```python
from build123d import *

# Parameters (mm, degrees)
SKETCH1_W           = 50.8
SKETCH1_H           = 304.8
BOSS_EXTRUDE1_DEPTH = 6.35
SKETCH2_R           = 3.429
CUT_EXTRUDE1_DEPTH  = 310.0695755


with BuildPart() as part:
    # Sketch1 → Boss-Extrude1 (new body)
    with BuildSketch(Plane.XY):
        with Locations((25.4, -152.4)):
            Rectangle(SKETCH1_W, SKETCH1_H)
    extrude(amount=BOSS_EXTRUDE1_DEPTH)

    # Sketch2 → Cut-Extrude1 (cut, through all)
    with BuildSketch(Plane.XY):
        with Locations((6.35, -6.35)):
            Circle(SKETCH2_R)
        with Locations((19.05, -6.35)):
            Circle(SKETCH2_R)
        with Locations((31.75, -6.35)):
            Circle(SKETCH2_R)
        with Locations((44.45, -6.35)):
            Circle(SKETCH2_R)
        with Locations((19.05, -19.05)):
            Circle(SKETCH2_R)
        with Locations((31.75, -19.05)):
            Circle(SKETCH2_R)
        with Locations((44.45, -19.05)):
            Circle(SKETCH2_R)
        with Locations((19.05, -31.75)):
            Circle(SKETCH2_R)
        with Locations((31.75, -31.75)):
            Circle(SKETCH2_R)
        with Locations((44.45, -31.75)):
            Circle(SKETCH2_R)
        with Locations((19.05, -44.45)):
            Circle(SKETCH2_R)
        with Locations((31.75, -44.45)):
            Circle(SKETCH2_R)
        with Locations((44.45, -44.45)):
            Circle(SKETCH2_R)
        with Locations((19.05, -57.15)):
            Circle(SKETCH2_R)
        with Locations((31.75, -57.15)):
            Circle(SKETCH2_R)
        with Locations((44.45, -57.15)):
            Circle(SKETCH2_R)
        with Locations((19.05, -69.85)):
            Circle(SKETCH2_R)
        with Locations((31.75, -69.85)):
            Circle(SKETCH2_R)
        with Locations((44.45, -69.85)):
            Circle(SKETCH2_R)
        with Locations((19.05, -82.55)):
            Circle(SKETCH2_R)
        with Locations((31.75, -82.55)):
            Circle(SKETCH2_R)
        with Locations((44.45, -82.55)):
            Circle(SKETCH2_R)
        with Locations((19.05, -95.25)):
            Circle(SKETCH2_R)
        with Locations((31.75, -95.25)):
            Circle(SKETCH2_R)
        with Locations((44.45, -95.25)):
            Circle(SKETCH2_R)
        with Locations((19.05, -107.95)):
            Circle(SKETCH2_R)
        with Locations((31.75, -107.95)):
            Circle(SKETCH2_R)
        with Locations((44.45, -107.95)):
            Circle(SKETCH2_R)
        with Locations((19.05, -120.65)):
            Circle(SKETCH2_R)
        with Locations((31.75, -120.65)):
            Circle(SKETCH2_R)
        with Locations((44.45, -120.65)):
            Circle(SKETCH2_R)
        with Locations((19.05, -133.35)):
            Circle(SKETCH2_R)
        with Locations((31.75, -133.35)):
            Circle(SKETCH2_R)
        with Locations((44.45, -133.35)):
            Circle(SKETCH2_R)
        with Locations((19.05, -146.05)):
            Circle(SKETCH2_R)
        with Locations((31.75, -146.05)):
            Circle(SKETCH2_R)
        with Locations((44.45, -146.05)):
            Circle(SKETCH2_R)
        with Locations((19.05, -158.75)):
            Circle(SKETCH2_R)
        with Locations((31.75, -158.75)):
            Circle(SKETCH2_R)
        with Locations((44.45, -158.75)):
            Circle(SKETCH2_R)
        with Locations((19.05, -171.45)):
            Circle(SKETCH2_R)
        with Locations((31.75, -171.45)):
            Circle(SKETCH2_R)
        with Locations((44.45, -171.45)):
            Circle(SKETCH2_R)
        with Locations((19.05, -184.15)):
            Circle(SKETCH2_R)
        with Locations((31.75, -184.15)):
            Circle(SKETCH2_R)
        with Locations((44.45, -184.15)):
            Circle(SKETCH2_R)
        with Locations((19.05, -196.85)):
            Circle(SKETCH2_R)
        with Locations((31.75, -196.85)):
            Circle(SKETCH2_R)
        with Locations((44.45, -196.85)):
            Circle(SKETCH2_R)
        with Locations((19.05, -209.55)):
            Circle(SKETCH2_R)
        with Locations((31.75, -209.55)):
            Circle(SKETCH2_R)
        with Locations((44.45, -209.55)):
            Circle(SKETCH2_R)
        with Locations((19.05, -222.25)):
            Circle(SKETCH2_R)
        with Locations((31.75, -222.25)):
            Circle(SKETCH2_R)
        with Locations((44.45, -222.25)):
            Circle(SKETCH2_R)
        with Locations((19.05, -234.95)):
            Circle(SKETCH2_R)
        with Locations((31.75, -234.95)):
            Circle(SKETCH2_R)
        with Locations((44.45, -234.95)):
            Circle(SKETCH2_R)
        with Locations((19.05, -247.65)):
            Circle(SKETCH2_R)
        with Locations((31.75, -247.65)):
            Circle(SKETCH2_R)
        with Locations((44.45, -247.65)):
            Circle(SKETCH2_R)
        with Locations((19.05, -260.35)):
            Circle(SKETCH2_R)
        with Locations((31.75, -260.35)):
            Circle(SKETCH2_R)
        with Locations((44.45, -260.35)):
            Circle(SKETCH2_R)
        with Locations((19.05, -273.05)):
            Circle(SKETCH2_R)
        with Locations((31.75, -273.05)):
            Circle(SKETCH2_R)
        with Locations((44.45, -273.05)):
            Circle(SKETCH2_R)
        with Locations((19.05, -285.75)):
            Circle(SKETCH2_R)
        with Locations((31.75, -285.75)):
            Circle(SKETCH2_R)
        with Locations((44.45, -285.75)):
            Circle(SKETCH2_R)
        with Locations((19.05, -298.45)):
            Circle(SKETCH2_R)
        with Locations((31.75, -298.45)):
            Circle(SKETCH2_R)
        with Locations((44.45, -298.45)):
            Circle(SKETCH2_R)
        with Locations((19.05, -311.15)):
            Circle(SKETCH2_R)
        with Locations((31.75, -311.15)):
            Circle(SKETCH2_R)
        with Locations((44.45, -311.15)):
            Circle(SKETCH2_R)
        with Locations((19.05, -323.85)):
            Circle(SKETCH2_R)
        with Locations((31.75, -323.85)):
            Circle(SKETCH2_R)
        with Locations((44.45, -323.85)):
            Circle(SKETCH2_R)
        with Locations((19.05, -336.55)):
            Circle(SKETCH2_R)
        with Locations((31.75, -336.55)):
            Circle(SKETCH2_R)
        with Locations((44.45, -336.55)):
            Circle(SKETCH2_R)
        with Locations((19.05, -349.25)):
            Circle(SKETCH2_R)
        with Locations((31.75, -349.25)):
            Circle(SKETCH2_R)
        with Locations((44.45, -349.25)):
            Circle(SKETCH2_R)
        with Locations((19.05, -361.95)):
            Circle(SKETCH2_R)
        with Locations((31.75, -361.95)):
            Circle(SKETCH2_R)
        with Locations((44.45, -361.95)):
            Circle(SKETCH2_R)
        with Locations((19.05, -374.65)):
            Circle(SKETCH2_R)
        with Locations((31.75, -374.65)):
            Circle(SKETCH2_R)
        with Locations((44.45, -374.65)):
            Circle(SKETCH2_R)
        with Locations((6.35, -19.05)):
            Circle(SKETCH2_R)
        with Locations((6.35, -31.75)):
            Circle(SKETCH2_R)
        with Locations((6.35, -44.45)):
            Circle(SKETCH2_R)
        with Locations((6.35, -57.15)):
            Circle(SKETCH2_R)
        with Locations((6.35, -69.85)):
            Circle(SKETCH2_R)
        with Locations((6.35, -82.55)):
            Circle(SKETCH2_R)
        with Locations((6.35, -95.25)):
            Circle(SKETCH2_R)
        with Locations((6.35, -107.95)):
            Circle(SKETCH2_R)
        with Locations((6.35, -120.65)):
            Circle(SKETCH2_R)
        with Locations((6.35, -133.35)):
            Circle(SKETCH2_R)
        with Locations((6.35, -146.05)):
            Circle(SKETCH2_R)
        with Locations((6.35, -158.75)):
            Circle(SKETCH2_R)
        with Locations((6.35, -171.45)):
            Circle(SKETCH2_R)
        with Locations((6.35, -184.15)):
            Circle(SKETCH2_R)
        with Locations((6.35, -196.85)):
            Circle(SKETCH2_R)
        with Locations((6.35, -209.55)):
            Circle(SKETCH2_R)
        with Locations((6.35, -222.25)):
            Circle(SKETCH2_R)
        with Locations((6.35, -234.95)):
            Circle(SKETCH2_R)
        with Locations((6.35, -247.65)):
            Circle(SKETCH2_R)
        with Locations((6.35, -260.35)):
            Circle(SKETCH2_R)
        with Locations((6.35, -273.05)):
            Circle(SKETCH2_R)
        with Locations((6.35, -285.75)):
            Circle(SKETCH2_R)
        with Locations((6.35, -298.45)):
            Circle(SKETCH2_R)
        with Locations((6.35, -311.15)):
            Circle(SKETCH2_R)
        with Locations((6.35, -323.85)):
            Circle(SKETCH2_R)
        with Locations((6.35, -336.55)):
            Circle(SKETCH2_R)
        with Locations((6.35, -349.25)):
            Circle(SKETCH2_R)
        with Locations((6.35, -361.95)):
            Circle(SKETCH2_R)
        with Locations((6.35, -374.65)):
            Circle(SKETCH2_R)
    extrude(amount=CUT_EXTRUDE1_DEPTH, mode=Mode.SUBTRACT)


solid = part.part
```
Check sheet for the modelled part. Datum: model origin and axes. Units: mm. Round coordinates to 2 decimals unless told otherwise and drop trailing zeros. Loops run counter-clockwise (first coordinate to the right, second up) from the corner with the lowest first, then second, coordinate; pieces in that order, holes last. Notation, with made-up numbers: M 87,88.5 L 136,88.5 A14 cw 136,92.5 Z; hole C 77,35 d6. An arc over 180 degrees is marked long. Answer as a JSON object with one key per item and string values.
1. Section check A-A (y = -273.05). Record the boundary of the cut face in (x, z).
Reply:
{"outline": "M 0,0 L 2.92,0 L 2.92,6.35 L 0,6.35 Z; M 9.78,0 L 15.62,0 L 15.62,6.35 L 9.78,6.35 Z; M 22.48,0 L 28.32,0 L 28.32,6.35 L 22.48,6.35 Z; M 35.18,0 L 41.02,0 L 41.02,6.35 L 35.18,6.35 Z; M 47.88,0 L 50.8,0 L 50.8,6.35 L 47.88,6.35 Z"}
2. Scan lines: line 1 (X direction, y = -222.25, z = 1.5); line 2 (X direction, y = -19.5, z = 5). Record each from-to range of solid material in increasing order.
Reply:
{"line 1": "x = 0 to 2.92, 9.78 to 15.62, 22.48 to 28.32, 35.18 to 41.02, 47.88 to 50.8", "line 2": "x = 0 to 2.95, 9.75 to 15.65, 22.45 to 28.35, 35.15 to 41.05, 47.85 to 50.8"}
3. Section check B-B (z = 4). State how many separate pieces and enclosed holes the cut face has, plus the area to 3 significant figures.
Reply:
{"separate pieces": "1", "enclosed holes": "96", "area": "11,900 mm²"}
